For this review, take the finished solid that the model builds, in its own axes (mm). Face numbers are marked on the shaded views. A direction names the side the tool comes from. Coordinates: 2 decimals unless noted, no trailing zeros. Loops run counter-clockwise (first coordinate to the right, second up) from the corner with the lowest first, then second, coordinate; pieces in that order, holes last. Notation, with made-up numbers: M -5.5,86 L 28.5,86 A11 cw 28.5,104 Z; hole C -17.75,64.25 d9. An arc over 180 degrees is marked long. Write item = value, one per line.
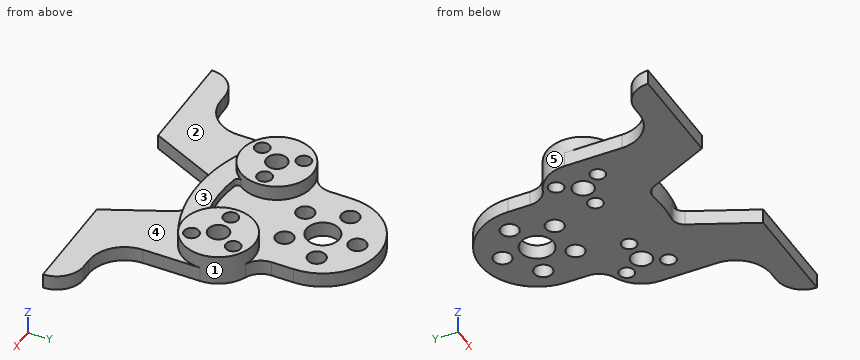
from build123d import *

# Parameters (mm, degrees)
EXTRUDE_1_DEPTH   = 10
EXTRUDE_1_2_DEPTH = 10
SKETCH_1_R        = 6
SKETCH_1_R_2      = 11
EXTRUDE_1_3_DEPTH = 10
EXTRUDE_2_DEPTH   = 15
SKETCH_1_4_R      = 24
SKETCH_1_4_R_2    = 5
SKETCH_1_4_R_3    = 7
EXTRUDE_3_DEPTH   = 20


with BuildPart() as part:
    # Sketch 1 → Extrude 1 (new body)
    with BuildSketch(Plane.XY):
        with BuildLine():
            Line((62, -38), (62, 0))
            ThreePointArc((62, 0), (58.784609691, -12), (50, -20.784609691))
            ThreePointArc((50, -20.784609691), (31.730847168, -29.014307175), (12.187732979, -33.436586413))
            ThreePointArc((12.187732979, -33.436586413), (17.041200429, -34.37997452), (20.413213913, -37.996001687))
            Line((20.413213913, -37.996001687), (40, -80))
            Line((40, -80), (110, -80))
            ThreePointArc((110, -80), (104.727922061, -67.272077939), (92, -62))
            Line((92, -62), (86, -62))
            ThreePointArc((86, -62), (69.029437252, -54.970562748), (62, -38))
        make_face()
    extrude(amount=EXTRUDE_1_DEPTH)



with BuildPart() as body_2:
    # Sketch 1 → Extrude 1 2 (new body)
    with BuildSketch(Plane.XY):
        with BuildLine():
            ThreePointArc((-50, -20.784609691), (-58.784609691, -12), (-62, 0))
            Line((-62, 0), (-62, -38))
            ThreePointArc((-62, -38), (-69.029437252, -54.970562748), (-86, -62))
            Line((-86, -62), (-92, -62))
            ThreePointArc((-92, -62), (-104.727922061, -67.272077939), (-110, -80))
            Line((-110, -80), (-40, -80))
            Line((-40, -80), (-20.413213913, -37.996001687))
            ThreePointArc((-20.413213913, -37.996001687), (-17.041200429, -34.37997452), (-12.187732979, -33.436586413))
            ThreePointArc((-12.187732979, -33.436586413), (-31.730847168, -29.014307175), (-50, -20.784609691))
        make_face()
    extrude(amount=EXTRUDE_1_2_DEPTH)


with BuildPart() as body_3:
    # Sketch 1 → Extrude 1 3 (new body)
    with BuildSketch(Plane.XY):
        with BuildLine():
            ThreePointArc((38, 50), (0, 88), (-38, 50))
            Line((-38, 50), (-38, 35.327043465))
            ThreePointArc((-38, 35.327043465), (-40.419617314, 27.459722648), (-46.842105263, 22.311816925))
            ThreePointArc((-46.842105263, 22.311816925), (-24.513164313, 19.852084605), (-14, 0))
            ThreePointArc((-14, 0), (-15.090152654, -7.151146382), (-18.261574548, -13.652639329))
            ThreePointArc((-18.261574548, -13.652639329), (-18.523440421, -16.011324994), (-16.696563974, -17.526083803))
            ThreePointArc((-16.696563974, -17.526083803), (0, -19.182069312), (16.696563974, -17.526083803))
            ThreePointArc((16.696563974, -17.526083803), (18.523440421, -16.011324994), (18.261574548, -13.652639329))
            ThreePointArc((18.261574548, -13.652639329), (19.210562093, 14.931745483), (46.842105263, 22.311816925))
            ThreePointArc((46.842105263, 22.311816925), (40.419617314, 27.459722648), (38, 35.327043465))
            Line((38, 35.327043465), (38, 50))
        make_face()
        with Locations((-13.519060803, 31.392609129)):
            Circle(SKETCH_1_R, mode=Mode.SUBTRACT)
        with Locations((0, 50)):
            Circle(SKETCH_1_R_2, mode=Mode.SUBTRACT)
        with Locations((-21.874299875, 57.107390871)):
            Circle(SKETCH_1_R, mode=Mode.SUBTRACT)
        with Locations((0, 73)):
            Circle(SKETCH_1_R, mode=Mode.SUBTRACT)
        with Locations((13.519060803, 31.392609129)):
            Circle(SKETCH_1_R, mode=Mode.SUBTRACT)
        with Locations((21.874299875, 57.107390871)):
            Circle(SKETCH_1_R, mode=Mode.SUBTRACT)
    extrude(amount=EXTRUDE_1_3_DEPTH)


with BuildPart() as part_1:
    add(part.part)

    add(body_2.part)  # Extrude 2 merges body 2

    add(body_3.part)  # Extrude 2 merges body 3
    # Sketch 1_3 → Extrude 2 (add)
    with BuildSketch(Plane.XY):
        with BuildLine():
            ThreePointArc((-16.696563974, -17.526083803), (-18.523440421, -16.011324994), (-18.261574548, -13.652639329))
            ThreePointArc((-18.261574548, -13.652639329), (-32.738150759, -23.416082989), (-50, -20.784609691))
            ThreePointArc((-50, -20.784609691), (-31.730847168, -29.014307175), (-12.187732979, -33.436586413))
            ThreePointArc((-12.187732979, -33.436586413), (0, -34.182069312), (12.187732979, -33.436586413))
            ThreePointArc((12.187732979, -33.436586413), (31.730847168, -29.014307175), (50, -20.784609691))
            ThreePointArc((50, -20.784609691), (32.738150759, -23.416082989), (18.261574548, -13.652639329))
            ThreePointArc((18.261574548, -13.652639329), (18.523440421, -16.011324994), (16.696563974, -17.526083803))
            ThreePointArc((16.696563974, -17.526083803), (0, -19.182069312), (-16.696563974, -17.526083803))
        make_face()
    extrude(amount=EXTRUDE_2_DEPTH)

    # Sketch 1_4 → Extrude 3 (add)
    # profile 1 of 2: a face of its own
    with BuildSketch(Plane.XY):
        with Locations(Location((-38, 0, 0), (0, 0, 180))):
            Circle(SKETCH_1_4_R)
        with Locations((-46, 13.856406461)):
            Circle(SKETCH_1_4_R_2, mode=Mode.SUBTRACT)
        with Locations((-46, -13.856406461)):
            Circle(SKETCH_1_4_R_2, mode=Mode.SUBTRACT)
        with Locations((-22, 0)):
            Circle(SKETCH_1_4_R_2, mode=Mode.SUBTRACT)
        with Locations((-38, 0)):
            Circle(SKETCH_1_4_R_3, mode=Mode.SUBTRACT)
    # profile 2 of 2: a face of its own
    with BuildSketch(Plane.XY):
        with Locations((38, 0)):
            Circle(SKETCH_1_4_R)
        with Locations((22, 0)):
            Circle(SKETCH_1_4_R_2, mode=Mode.SUBTRACT)
        with Locations((46, 13.856406461)):
            Circle(SKETCH_1_4_R_2, mode=Mode.SUBTRACT)
        with Locations((46, -13.856406461)):
            Circle(SKETCH_1_4_R_2, mode=Mode.SUBTRACT)
        with Locations((38, 0)):
            Circle(SKETCH_1_4_R_3, mode=Mode.SUBTRACT)
    extrude(amount=EXTRUDE_3_DEPTH)


solid = part_1.part
Q1. Add section A-A (z = 17.75). State how many separate pieces and enclosed holes the cut face has, and give its area (3 significant figures).
Solved:
separate_pieces = 2
enclosed_holes = 8
area = 2,840 mm²
Q2. Draft analysis for pull direction X (two halves, no side actions). For the marked faces 4 and 5, state which applies: +X half, -X half, draft (parallel to the pull), parting line (faces both ways), or undercut.
Solved:
face_4 = draft
face_5 = undercut
Q3. For line 1 along Y through (x, z) = (0, 7.5); line 2 along X through (y, z) = (53.5, 1.75); line 3 along X through (y, z) = (-17.5, 6.5), list the stretches that pass through material, from the lowest coordinate up.
Solved:
line_1 = -34.18 to 39, 61 to 67, 79 to 88
line_2 = -37.84 to -26.67, -17.08 to -10.43, 10.43 to 17.08, 26.67 to 37.84
line_3 = -62 to -49.42, -42.58 to 42.58, 49.42 to 62
Q4. Machinability: for the marked faces 1, 2 and 3, which of the approach directions +Z, -Z, +X, -X, +Y, -Y give a long, thin tool a straight path to every point of the face, cutting with its end or side? Answer none if there is none.
Solved:
face_1 = +Z
face_2 = +Z, -X, -Y
face_3 = +Z, -Y
Q5. For pin 1 Ø1 at (y, z) = (41, 2.5) entering from +X; pin 2 Ø5 at (x, z) = (-46, 17) entering from +Y; pin 3 Ø2 at (y, z) = (4.5, 11) entering from -X; pin 4 Ø9 at (x, y) = (-46, 13.86) entering from +Z, all flat-tipped, find the tip position at first contact; note any pin that passes through.
Solved:
pin_1 = 38
pin_2 = 23.36
pin_3 = -61.74
pin_4 = through
Q6. Add section B-B (x = 96). Write out the cut boundary in (y, z).
Solved:
outline = M -80,0 L -62.45,0 L -62.45,10 L -80,10 Z
